```python
from build123d import *

# Parameters (mm, degrees)
SKETCH1_R           = 38.1
SKETCH1_R_2         = 6.35
BOSS_EXTRUDE1_DEPTH = 25.4
CUT_EXTRUDE1_DEPTH  = 19.05
SKETCH3_R           = 4.191
CUT_EXTRUDE2_DEPTH  = 144.195909909
FILLET1_R           = 7.62
FILLET2_R           = 5.08


with BuildPart() as part:
    # Sketch1 → Boss-Extrude1 (new body)
    with BuildSketch(Plane.XY):
        Polygon((-15.376904817, 111.859177573), (19.281255226, 111.859177573), (19.281255226, 51.662487547), (85.717168685, 13.57632424), (54.880053148, -63.203130515), (31.826573213, -53.944106385), (13.090387594, -70.609161185), (13.090387594, -83.309161185), (-15.546461726, -83.309161185), (-15.546461726, -68.356164498), (-49.113541671, -12.382140744), (-84.5631354, -12.382140744), (-84.5631354, 11.598068918), (-43.284636092, 11.598068918), align=None)
        Circle(SKETCH1_R, mode=Mode.SUBTRACT)
        with Locations((0, 99.159177573)):
            Circle(SKETCH1_R_2, mode=Mode.SUBTRACT)
        with Locations((-2.02148369, -70.609161185)):
            Circle(SKETCH1_R_2, mode=Mode.SUBTRACT)
        with Locations((-71.8631354, 0)):
            Circle(SKETCH1_R_2, mode=Mode.SUBTRACT)
    extrude(amount=BOSS_EXTRUDE1_DEPTH)

    # Sketch2 → Cut-Extrude1 (cut)
    with BuildSketch(Plane.XY.offset(25.4)):
        Polygon((445.884060036, -192.898973947), (85.717168685, 13.57632424), (66.538177491, 24.571193621), (31.826573213, -53.944106385), (-136.039422118, -433.645628635), (181.37430947, -1200.885797388), (763.297791624, -960.1391427), align=None)
    extrude(amount=-CUT_EXTRUDE1_DEPTH, mode=Mode.SUBTRACT)

    # Sketch3 → Cut-Extrude2 (cut, through all)
    with BuildSketch(Plane.XY.offset(25.4)):
        with Locations((71.679164996, 8.361848351)):
            Circle(SKETCH3_R)
        with Locations((49.148937242, -47.734792738)):
            Circle(SKETCH3_R)
    extrude(amount=-CUT_EXTRUDE2_DEPTH, mode=Mode.SUBTRACT)

    # Fillet1
    fillet1_edges = [part.edges().sort_by_distance(p)[0] for p in [
        (13.090387594, -70.609161185, 12.7),
        (13.090387594, -83.309161185, 12.7),
        (-15.546461726, -83.309161185, 12.7),
        (-15.546461726, -68.356164498, 12.7),
        (-49.113541671, -12.382140744, 12.7),
        (-84.5631354, -12.382140744, 12.7),
        (-84.5631354, 11.598068918, 12.7),
        (-43.284636092, 11.598068918, 12.7),
        (-15.376904817, 111.859177573, 12.7),
        (19.281255226, 111.859177573, 12.7),
        (19.281255226, 51.662487547, 12.7),
        (66.538177491, 24.571193621, 15.875),
    ]]
    fillet(fillet1_edges, radius=FILLET1_R)

    # Fillet2
    fillet2_edges = [part.edges().sort_by_distance(p)[0] for p in [
        (85.717168685, 13.57632424, 3.175),
        (54.880053148, -63.203130515, 3.175),
        (31.826573213, -53.944106385, 3.175),
    ]]
    fillet(fillet2_edges, radius=FILLET2_R)


solid = part.part
```
Geometry check sheet. Reference: the model listing, model coordinates, mm. A direction names the side the tool comes from. Coordinates: 2 decimals unless noted, no trailing zeros. Write each loop counter-clockwise with the first axis right and the second up, starting at its lowest first coordinate (ties: lowest second). Pieces come first, ordered by that corner, then holes. Notation, with made-up numbers: M -1.5,1.25 L 52.5,1.25 A6 ccw 52.5,9.25 Z; hole C 15,83 d7. An arc over 180 degrees is marked long. One line per item, written item: value. Start each with the question number.
(1) Sectioned sample at A-A, the plane y = -19. Enter the section's corners in (x, z).
(2) Sectioned sample at B-B, the plane z = 15. State how many separate pieces and enclosed holes the cut face has, and give its area (3 significant figures).
(3) Tool access check on faces 5 (the face through (42.564, -58.257, 3.131)), 6 (the face through (19.281, 80, 13)), 7 (the face through (48.02, -17.32, 16.01)), 8 (the face through (-63, 11.598, 13)), 9 (the face through (-13.37, -81.02, 12.88)). Record the directions out of +Z, -Z, +X, -X, +Y, -Y that give a thin tool (end or side, any length) a straight path to the whole face; none if there is none.
(4) Scan lines: line 1 along Y through (x, z) = (0, 6.5); line 2 along Y through (x, z) = (34.5, 11.75); line 3 along Y through (x, z) = (-61.5, 3.75). Record each from-to range of solid material in increasing order. Write a range as [from, to].
(5) Sectioned sample at C-C, the plane x = 0. Enter the section's corners in (y, z).
(6) Depth check by flat-ended pin: pin 1 (13.5 mm diameter, centred on x = 71.68, y = 8.36, fed in from +Z); pin 2 (8 mm diameter, centred on x = 57.5, z = 11, fed in from +Y); pin 3 (1.3 mm diameter, centred on y = -75, z = 9.5, fed in from +X); pin 4 (14.5 mm diameter, centred on x = 0, y = 99.16, fed in from -Z). Enter the tip coordinate at first touch or a pass-through.
(7) Release check for a two-part mould opening along Y. For faces 1 (the face through (-84.563, 0, 13)), 2 (the face through (-49.722, -13.345, 12.878)), 3 (the face through (45.555, 36.6, 12.522)), 4 (the face through (-2.848, -64.313, 12.522)) record: released by +Y, released by -Y, zero draft, split by the parting line, or undercut.
Filled sheet:
1. outline: M -45.14,0 L -33.02,0 L -33.02,25.4 L -45.14,25.4 Z; M 33.02,0 L 72.63,0 L 72.63,6.35 L 47.28,6.35 L 47.28,25.4 L 33.02,25.4 Z
2. separate pieces: 1
2. enclosed holes: 4
2. area: 8,730 mm²
3. face 5: +Z, -Z, -Y
3. face 6: +Z, -Z, +X, +Y
3. face 7: +Z, +X, -Y
3. face 8: +Z, -Z, -X, +Y
3. face 9: +Z, -Z, -X, -Y
4. line 1: [-83.31, -76.63], [-64.59, -38.1], [38.1, 92.81], [105.51, 111.86]
4. line 2: [-47.9, -16.17], [16.17, 42.94]
4. line 3: [-12.38, 11.6]
5. outline: M -83.31,0 L -76.63,0 L -76.63,25.4 L -83.31,25.4 Z; M -64.59,0 L -38.1,0 L -38.1,25.4 L -64.59,25.4 Z; M 38.1,0 L 92.81,0 L 92.81,25.4 L 38.1,25.4 Z; M 105.51,0 L 111.86,0 L 111.86,25.4 L 105.51,25.4 Z
6. pin 1: z = 6.35
6. pin 2: y = 32.05
6. pin 3: x = 13.09
6. pin 4: z = 0
7. face 1: zero draft
7. face 2: released by -Y
7. face 3: released by +Y
7. face 4: undercut
